```python
from build123d import *

# Parameters (mm, degrees)
BOSS_EXTRUDE1_DEPTH     = 40.6
CUT_EXTRUDE1_DEPTH      = 81.783971182
CUT_EXTRUDE1_DEPTH_BACK = 81.783971182
SKETCH2_R               = 1.5
CUT_EXTRUDE2_DEPTH      = 81.775305632
CUT_EXTRUDE2_DEPTH_BACK = 81.775305632
SKETCH3_R               = 1.5


with BuildPart() as part:
    # Sketch1 → Boss-Extrude1 (new body)
    with BuildSketch(Plane(origin=(0, 0, 0), x_dir=(1, 0, 0), z_dir=(0, 1, 0))):
        Polygon((0, 0), (0, 51), (3.5, 51), (3.5, 3.5), (51.2, 3.5), (51.2, 0), align=None)
    extrude(amount=BOSS_EXTRUDE1_DEPTH)

    # Sketch2 → Cut-Extrude1 (cut, two sides: drawn at the far end of the back side and taken through both)
    with BuildSketch(Plane(origin=(0, 0, -3.5), x_dir=(-1, 0, 0), z_dir=(0, 0, -1)).offset(-CUT_EXTRUDE1_DEPTH_BACK)):
        with BuildLine():
            ThreePointArc((-10.3, 35.3), (-10.414180701, 35.874025149), (-10.739339828, 36.360660172))
            Line((-10.739339828, 36.360660172), (-12.860660172, 34.239339828))
            ThreePointArc((-12.860660172, 34.239339828), (-11.225974851, 33.914180701), (-10.3, 35.3))
        make_face()
        with BuildLine():
            Line((-12.860660172, 34.239339828), (-10.739339828, 36.360660172))
            ThreePointArc((-10.739339828, 36.360660172), (-12.860660172, 36.360660172), (-12.860660172, 34.239339828))
        make_face()
        with Locations((-41.8, 35.3)):
            Circle(SKETCH2_R)
        with BuildLine():
            ThreePointArc((-23.8, 20.3), (-24.028361402, 21.448050297), (-24.678679656, 22.421320344))
            Line((-24.678679656, 22.421320344), (-28.921320344, 18.178679656))
            ThreePointArc((-28.921320344, 18.178679656), (-25.651949703, 17.528361402), (-23.8, 20.3))
        make_face()
        with BuildLine():
            Line((-28.921320344, 18.178679656), (-24.678679656, 22.421320344))
            ThreePointArc((-24.678679656, 22.421320344), (-28.921320344, 22.421320344), (-28.921320344, 18.178679656))
        make_face()
        with Locations((-11.8, 5.3)):
            Circle(SKETCH2_R)
        with BuildLine():
            ThreePointArc((-40.3, 5.3), (-40.414180701, 5.874025149), (-40.739339828, 6.360660172))
            Line((-40.739339828, 6.360660172), (-42.860660172, 4.239339828))
            ThreePointArc((-42.860660172, 4.239339828), (-41.225974851, 3.914180701), (-40.3, 5.3))
        make_face()
        with BuildLine():
            Line((-42.860660172, 4.239339828), (-40.739339828, 6.360660172))
            ThreePointArc((-40.739339828, 6.360660172), (-42.860660172, 6.360660172), (-42.860660172, 4.239339828))
        make_face()
    extrude(amount=CUT_EXTRUDE1_DEPTH + CUT_EXTRUDE1_DEPTH_BACK, mode=Mode.SUBTRACT)

    # Sketch3 → Cut-Extrude2 (cut, two sides: drawn at the far end of the back side and taken through both)
    with BuildSketch(Plane(origin=(3.5, 0, 0), x_dir=(0, 0, -1), z_dir=(1, 0, 0)).offset(-CUT_EXTRUDE2_DEPTH_BACK)):
        with BuildLine():
            ThreePointArc((37, 32.8), (38.5, 31.3), (40, 32.8))
            Line((40, 32.8), (37, 32.8))
        make_face()
        with BuildLine():
            Line((37, 32.8), (40, 32.8))
            ThreePointArc((40, 32.8), (38.5, 34.3), (37, 32.8))
        make_face()
        with BuildLine():
            ThreePointArc((7, 32.8), (8.5, 31.3), (10, 32.8))
            Line((10, 32.8), (7, 32.8))
        make_face()
        with BuildLine():
            Line((7, 32.8), (10, 32.8))
            ThreePointArc((10, 32.8), (8.5, 34.3), (7, 32.8))
        make_face()
        with Locations((8.5, 7.8)):
            Circle(SKETCH3_R)
        with Locations((38.5, 7.8)):
            Circle(SKETCH3_R)
    extrude(amount=CUT_EXTRUDE2_DEPTH + CUT_EXTRUDE2_DEPTH_BACK, mode=Mode.SUBTRACT)


solid = part.part
```
Can you work these out from the model? Positions are in its coordinate system, mm. A direction names the side the tool comes from. Give positions to 0.01 mm unless a question says otherwise; leave off trailing zeros. Loops run counter-clockwise (first coordinate to the right, second up) from the corner with the lowest first, then second, coordinate; pieces in that order, holes last. Notation, with made-up numbers: M 39.25,58 L 43.25,58 A19 ccw 43.25,64 Z; hole C 7,-26.5 d5. An arc over 180 degrees is marked long. Use one line per item in the form item = value. Start each with the question number.
(1) I want a section at A-A, the plane y = 32.8. Write out the boundary of the cut face in (x, z).
(2) Please list where these lines run through material, in increasing order: line 1 (Y direction, x = 1.7, z = -38.5); line 2 (X direction, y = 5.3, z = -2.3); line 3 (Y direction, x = 41.8, z = -1.2).
(3) I want a section at C-C, the plane x = 34. Write out the boundary of the cut face in (y, z), and give its area (3 significant figures).
(4) On a 3-axis mill with a long thin cutter (end or side, diameter ignored), from which of +Z, -Z, +X, -X, +Y, -Y can I reach the whole of each face in a straight line? I mean faces 1 (the flat face through (0, 20, -25)), 2 (the flat face through (3.5, 20, -28)). Say none if no direction works.
(5) I'm going to push flat-ended pins straight in: P1, Ø1.8, axis at x = 11.8, y = 5.3, coming from the +Z side; P2, Ø20.5, axis at y = 13.5, z = -32, coming from the +X side; P3, Ø6, axis at x = 21, y = 35.5, coming from the -Z side. Where does each tip first touch, or does it pass through?
(6) Thinking about a two-plate mould opening in Y: for faces 3 (the flat face through (51.2, 20, -2)), 4 (the flat face through (14, 0, -3)), 5 (the cylindrical face through (1.73, 33.81, -37.39)), which applies, released by +Y, released by -Y, zero draft, split by the parting line, or undercut?
(7) I want a section at B-B, the plane z = -38.5. Write out the boundary of the cut face in (x, y).
(8) I want a section at D-D, the plane z = -9. Write out the boundary of the cut face in (x, y).
Worked out:
q1.outline = M 0,-51 L 3.5,-51 L 3.5,-40 L 0,-40 Z; M 0,-37 L 3.5,-37 L 3.5,-10 L 0,-10 Z; M 0,-7 L 3.5,-7 L 3.5,-3.5 L 51.2,-3.5 L 51.2,0 L 0,0 Z
q2.line_1 = 0 to 6.3, 9.3 to 31.3, 34.3 to 40.6
q2.line_2 = 0 to 10.3, 13.3 to 40.3, 43.3 to 51.2
q2.line_3 = 0 to 3.8, 6.8 to 33.8, 36.8 to 40.6
q3.outline = M 0,-3.5 L 40.6,-3.5 L 40.6,0 L 0,0 Z
q3.area = 142 mm²
q4.face_1 = +Z, -Z, -X, +Y, -Y
q4.face_2 = -Z, +X, +Y, -Y
q5.P1 = through
q5.P2 = 3.5
q5.P3 = -3.5
q6.face_3 = zero draft
q6.face_4 = released by -Y
q6.face_5 = undercut
q7.outline = M 0,0 L 3.5,0 L 3.5,6.3 L 0,6.3 Z; M 0,9.3 L 3.5,9.3 L 3.5,31.3 L 0,31.3 Z; M 0,34.3 L 3.5,34.3 L 3.5,40.6 L 0,40.6 Z
q8.outline = M 0,0 L 3.5,0 L 3.5,6.39 L 0,6.39 Z; M 0,9.21 L 3.5,9.21 L 3.5,31.39 L 0,31.39 Z; M 0,34.21 L 3.5,34.21 L 3.5,40.6 L 0,40.6 Z
